Input: part model. Units: mm. Frame: model coordinates. Face numbers are marked on the shaded views. A direction names the side the tool comes from. Round coordinates to 2 decimals unless told otherwise and drop trailing zeros. Order: outer loops, then holes, each group sorted by start corner. A loop starts at its lowest first (then second) coordinate and runs counter-clockwise, first axis right, second up. Notation, with made-up numbers: (-40, 32.5) -> (-27, 32.5) arc R31 ccw to (-27, 69.5) -> close; hole circle Ø10 at (51, -21). An arc over 180 degrees is marked (long way). Use a Markdown table: item, result.
from build123d import *

# Parameters (mm, degrees)
SKETCH1_W                = 250
SKETCH1_H                = 250
BOSS_EXTRUDE1_DEPTH      = 10
SKETCH2_R                = 15
CUT_EXTRUDE1_DEPTH       = 10
SKETCH3_W                = 125
SKETCH3_H                = 10
BOSS_EXTRUDE2_DEPTH      = 250
BOSS_EXTRUDE3_DEPTH      = 10
BOSS_EXTRUDE4_DEPTH      = 10
BOSS_EXTRUDE4_DEPTH_BACK = 10


with BuildPart() as part:
    # Sketch1 → Boss-Extrude1 (new body)
    with BuildSketch(Plane.XY):
        with Locations((28.899957468, -24.872643547)):
            Rectangle(SKETCH1_W, SKETCH1_H)
    extrude(amount=BOSS_EXTRUDE1_DEPTH)

    # Sketch2 → Cut-Extrude1 (cut)
    with BuildSketch(Plane.XY.offset(10)):
        with Locations((-71.100042532, 75.127356453)):
            Circle(SKETCH2_R)
        with Locations((128.899957468, 75.127356453)):
            Circle(SKETCH2_R)
        with Locations((128.899957468, -124.872643547)):
            Circle(SKETCH2_R)
        with Locations((-71.100042532, -124.872643547)):
            Circle(SKETCH2_R)
    extrude(amount=-CUT_EXTRUDE1_DEPTH, mode=Mode.SUBTRACT)

    # Sketch3 → Boss-Extrude2 (add)
    with BuildSketch(Plane.ZY.offset(96.100042532)):
        with Locations((72.5, -29.872643547)):
            Rectangle(SKETCH3_W, SKETCH3_H)
    extrude(amount=-BOSS_EXTRUDE2_DEPTH)

    # Sketch4 → Boss-Extrude3 (add)
    with BuildSketch(Plane.ZY.offset(71.100042532)):
        Polygon((72.5, -34.872643547), (10, -92.372643547), (10, -34.872643547), align=None)
    boss_extrude3 = extrude(amount=BOSS_EXTRUDE3_DEPTH)

    # Mirror1: Boss-Extrude3 across plane
    add(boss_extrude3.mirror(Plane.ZY.offset(-28.899957468)))

    # Sketch5 → Boss-Extrude4 (add, two sides)
    with BuildSketch(Plane.ZY.offset(-28.899957468)) as boss_extrude4_sk:
        with BuildLine():
            ThreePointArc((75.620200175, -34.872643547), (72.713276092, -35.419470238), (70.203747928, -36.985195453))
            Line((70.203747928, -36.985195453), (12.583547753, -89.995779614))
            ThreePointArc((12.583547753, -89.995779614), (10.67430488, -92.668544051), (10, -95.883227708))
            Line((10, -95.883227708), (10, -34.872643547))
            Line((10, -34.872643547), (75.620200175, -34.872643547))
        make_face()
    extrude(amount=BOSS_EXTRUDE4_DEPTH)
    extrude(boss_extrude4_sk.sketch, amount=-BOSS_EXTRUDE4_DEPTH_BACK)


solid = part.part
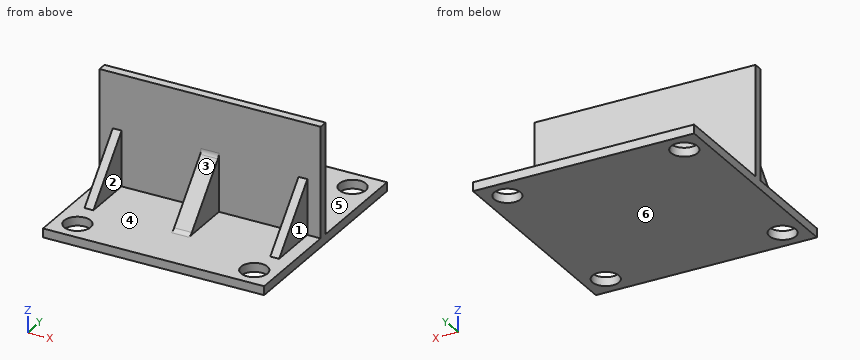
1) Cut plane C-C on y = -121.5. Return loops of the section in (x, z).
Answer key:
| item | result |
|---|---|
| outline | (-96.1, 0) -> (-85.72, 0) -> (-85.72, 10) -> (-96.1, 10) -> close; (-56.48, 0) -> (114.28, 0) -> (114.28, 10) -> (-56.48, 10) -> close; (143.52, 0) -> (153.9, 0) -> (153.9, 10) -> (143.52, 10) -> close |
2) Ray query, probe 1 along X at (y, z) = (-53.5, 28); probe 2 along X at (y, z) = (-119, 8); probe 3 along Z at (x, y) = (46.5, 30.5). Return the intervals inside material, ascending.
Answer key:
| item | result |
|---|---|
| probe 1 | x = -81.1 to -71.1, 18.9 to 38.9, 128.9 to 138.9 |
| probe 2 | x = -96.1 to -84.9, -57.3 to 115.1, 142.7 to 153.9 |
| probe 3 | z = 0 to 10 |
3) Set-up query: the marked faces 4, 5 and 6. Return all of +Z, -Z, +X, -X, +Y, -Y with unobstructed straight access to the full face (end or side cutting, diameter ignored); none if empty.
Answer key:
| item | result |
|---|---|
| face 4 | +Z, -Y |
| face 5 | +Z, +X, -X, +Y |
| face 6 | -Z, +X, -X, +Y, -Y |
4) Cut plane A-A on x = 134. Return loops of the section in (y, z).
Answer key:
| item | result |
|---|---|
| outline | (-149.87, 0) -> (-138.98, 0) -> (-138.98, 10) -> (-149.87, 10) -> close; (-110.77, 0) -> (61.02, 0) -> (61.02, 10) -> (-24.87, 10) -> (-24.87, 135) -> (-34.87, 135) -> (-34.87, 72.5) -> (-92.37, 10) -> (-110.77, 10) -> close; (89.23, 0) -> (100.13, 0) -> (100.13, 10) -> (89.23, 10) -> close |
5) Cut plane D-D on z = 62.5. Return loops of the section in (x, y), and give its area (3 significant figures).
Answer key:
| item | result |
|---|---|
| outline | (-96.1, -34.87) -> (-81.1, -34.87) -> (-81.1, -44.07) -> (-71.1, -44.07) -> (-71.1, -34.87) -> (18.9, -34.87) -> (18.9, -44.07) -> (38.9, -44.07) -> (38.9, -34.87) -> (128.9, -34.87) -> (128.9, -44.07) -> (138.9, -44.07) -> (138.9, -34.87) -> (153.9, -34.87) -> (153.9, -24.87) -> (-96.1, -24.87) -> close |
| area | 2,870 mm^2 |
6) Cut plane B-B on x = -30.5. Return loops of the section in (y, z), and give its area (3 significant figures).
Answer key:
| item | result |
|---|---|
| outline | (-149.87, 0) -> (100.13, 0) -> (100.13, 10) -> (-24.87, 10) -> (-24.87, 135) -> (-34.87, 135) -> (-34.87, 10) -> (-149.87, 10) -> close |
| area | 3,750 mm^2 |
7) Draft query along X for the marked faces 1, 2 and 3. Return one class per face: released by +X, released by -X, zero draft, split by the parting line, or undercut.
Answer key:
| item | result |
|---|---|
| face 1 | released by +X |
| face 2 | undercut |
| face 3 | zero draft |
8) Contact query for flat-ended pins moving along their axis: P1, Ø12, axis at x = -43, z = 54, coming from the +Y side; P2, Ø17, axis at y = -67.5, z = 55.5, coming from the +X side; P3, Ø8, axis at x = 80, z = 103, coming from the -Y side; P4, Ø17, axis at y = -58.5, z = 27, coming from the -X side. Output: stop coordinate, or through.
Answer key:
| item | result |
|---|---|
| P1 | stops at y = -24.87 |
| P2 | passes through |
| P3 | stops at y = -34.87 |
| P4 | stops at x = -81.1 |
